The listing builds one solid part. Answer for the finished solid, in the listing's coordinates (mm). Face numbers are marked on the shaded views. A direction names the side the tool comes from. Give positions to 0.01 mm unless a question says otherwise; leave off trailing zeros. Order: outer loops, then holes, each group sorted by start corner. A loop starts at its lowest first (then second) coordinate and runs counter-clockwise, first axis right, second up.
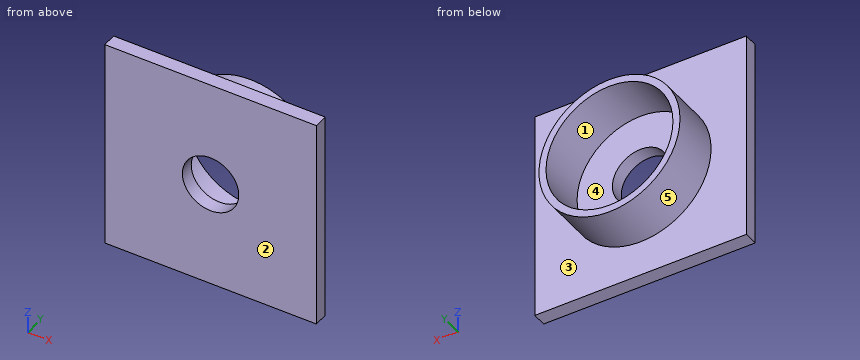
Autodesk Inventor part; units mm, degrees
ref_plane "YZ Plane" through (0, 0, 0) normal (1, 0, 0) x (0, 1, 0)
ref_plane "XZ Plane" through (0, 0, 0) normal (0, 1, 0) x (-1, 0, 0)
ref_plane "XY Plane" through (0, 0, 0) normal (0, 0, 1) x (1, 0, 0)
sketch "Boceto1" plane through (0, 0, 0) normal (0, 1, 0) x (-1, 0, 0)
  line L0 (15, -15) -> (-15, -15)
  line L1 (-15, -15) -> (-15, 15)
  line L2 (-15, 15) -> (15, 15)
  line L3 (15, 15) -> (15, -15)
  line L4 (15, -15) -> (-15, 15) construction
  line L5 (-15, -15) -> (15, 15) construction
  circle A0 centre (0, 0) radius 9
  circle A1 centre (0, 0) radius 4
  circle A2 centre (0, 0) radius 10
  dimension "d0" = 30
  dimension "d1" = 30
  dimension "d9" = 18
  dimension "d12" = 8
  dimension "d15" = 20
extrude "Extrusión1" add sketch "Boceto1" against normal blind 2 contours L0 L1 L2 L3 | A0 | A1 | A2
extrude "Extrusión4" cut sketch "Boceto1" against normal blind 3 contours A1
extrude "Extrusión5" add sketch "Boceto1" along normal blind 7 contours A2
properties part number "RodamientoAspa"
1) Straight lines are drawn through the part: probe 1 along Z at (x, y) = (0, 2.5); probe 2 along Y at (x, z) = (-6.75, 1); probe 3 along Z at (x, y) = (-1, 5.5). For each, find the intervals that lie inside material, in ascending order.
Geometry says:
probe 1: z = -10 to -9, 9 to 10
probe 2: y = -2 to 0
probe 3: z = -9.95 to -8.94, 8.94 to 9.95
2) A tool of negligible diameter and unlimited length cuts with its end or side. For the marked faces 1 and 2, from which of +Z, -Z, +X, -X, +Y, -Y can it reach the whole face along a straight path? Write none if from no direction.
Geometry says:
face 1: +Y
face 2: +Z, -Z, +X, -X, -Y
3) For a pull along X with two mould halves and no side action, classify the marked faces 3, 4 and 5 as +X half, -X half, draft (parallel to the pull), parting line (faces both ways), or undercut.
Geometry says:
face 3: draft
face 4: undercut
face 5: parting line
4) Find section B-B (x = 0). Write down the section's boundary in (y, z).
Geometry says:
outline: (-2, -15) - (0, -15) - (0, -10) - (7, -10) - (7, -9) - (0, -9) - (0, -4) - (-2, -4) - close; (-2, 4) - (0, 4) - (0, 9) - (7, 9) - (7, 10) - (0, 10) - (0, 15) - (-2, 15) - close
5) Find section C-C (y = 2.75). Write down the section's boundary in (x, z).
Geometry says:
outline: circle Ø20 at (0, 0); hole circle Ø18 at (0, 0)
6) Find section A-A (z = 0). Write down the section's boundary in (x, y), then the cut area to 3 significant figures.
Geometry says:
outline: (-15, -2) - (-4, -2) - (-4, 0) - (-9, 0) - (-9, 7) - (-10, 7) - (-10, 0) - (-15, 0) - close; (4, -2) - (15, -2) - (15, 0) - (10, 0) - (10, 7) - (9, 7) - (9, 0) - (4, 0) - close
area: 58.0 mm2
7) Find section D-D (x = 6). Write down the section's boundary in (y, z).
Geometry says:
outline: (-2, -15) - (0, -15) - (0, -8) - (7, -8) - (7, -6.71) - (0, -6.71) - (0, 6.71) - (7, 6.71) - (7, 8) - (0, 8) - (0, 15) - (-2, 15) - close
8) Given P1, Ø5, axis at x = 10.5, y = 4, coming from the +Z side; P2, Ø14.5, axis at x = 3.5, z = 3.5, coming from the +Y side; P3, Ø2, axis at x = 3.5, y = 3.5, coming from the +Z side; P4, Ø4, axis at y = 4.5, z = -8.5, coming from the +X side, each flat-ended and moving along its own axis, determine where each tip first touches the part or whether it passes through.
Geometry says:
P1: stops at z = 6
P2: stops at y = 7
P3: stops at z = 9.68
P4: stops at x = 7.6
